For this review, take the finished solid that the model builds, in its own axes (mm). A direction names the side the tool comes from. Round coordinates to 2 decimals unless told otherwise and drop trailing zeros. Write each loop counter-clockwise with the first axis right and the second up, starting at its lowest first coordinate (ties: lowest second). Pieces come first, ordered by that corner, then holes. Notation, with made-up numbers: (69.5, 58.5) -> (120.5, 58.5) arc R21 cw to (120.5, 74.5) -> close; hole circle Ø3 at (-15.5, -10). An arc over 180 degrees is marked (long way). Write each question's results on one line, items separated by ' | '. Start each with the question number.
Item 1: The part is to be moulded in two halves that separate along X. For faces 1 (the cylindrical face through (6.06, -27.1, 20.28)), 2 (the flat face through (-17.5, 102, 20)), 3 (the cylindrical face through (5, -33, 1)), say which applies: +X half, -X half, draft (parallel to the pull), parting line (faces both ways), or undercut.
Item 2: Clearance check with flat-ended pins moving along their axes: pin 1 (0.6 mm diameter, centred on x = 4.5, z = 6.5, fed in from -Y); pin 2 (6 mm diameter, centred on y = 94.5, z = 24.5, fed in from +X); pin 3 (9 mm diameter, centred on x = 9.5, y = -49, fed in from +Z); pin 4 (3 mm diameter, centred on x = 15.5, y = 67, fed in from +Z). State where each tip first meets the part, or that it passes through.
Item 3: Add section A-A (y = 16). State the section outline as (x, z) points.
Item 4: Tool access review of faces 4 (the cylindrical face through (12.52, -46.26, 25.57)), 5 (the flat face through (5.2, -39, 20)), 6 (the cylindrical face through (4.9, -25.86, 20.28)): name each direction out of +Z, -Z, +X, -X, +Y, -Y from which nothing blocks a thin tool from reaching the whole face with its end or side.
Item 5: To check wall thickness, follow line 1 along Y through (x, z) = (13.5, 9.5); line 2 along X through (y, z) = (66.5, 38); line 3 along Y through (x, z) = (-2, 35.5). State the ranges of each line that lie inside material, in increasing order.
Item 6: Add section B-B (x = -5). State the section outline as (y, z) points.
from build123d import *

# Parameters (mm, degrees)
PAD_DEPTH    = 40
PAD001_DEPTH = 7
FILLET_R     = 3
FILLET001_R  = 5


with BuildPart() as part:
    # Sketch → Pad (new body)
    with BuildSketch(Plane.XY):
        Polygon((-17.5, 114), (17.5, 114), (17.5, 0), (24, 0), (24, -25), (4, -25), (4, -35), (5.2, -35), (5.2, -26.2), (25.2, -26.2), (25.2, 1.2), (18.7, 1.2), (18.7, 115.2), (-18.7, 115.2), (-18.7, 94), (-17.5, 94), align=None)
    extrude(amount=PAD_DEPTH)

    # Sketch001 → Pad001 (join, symmetric)
    with BuildSketch(Plane.XY.offset(20)):
        with BuildLine():
            Line((4, -35), (4, -55))
            ThreePointArc((4, -55), (7.7, -58.233631), (11.4, -55))
            Line((13.4, -45), (11.4, -55))
            Line((12.292308, -44.538462), (13.4, -45))
            Line((10.2, -55), (12.292308, -44.538462))
            ThreePointArc((5.2, -55), (7.7, -57.04951), (10.2, -55))
            Line((5.2, -55), (5.2, -35))
            Line((5.2, -35), (4, -35))
        make_face()
    extrude(amount=PAD001_DEPTH, both=True)

    # Fillet
    fillet_edges = [part.edges().sort_by_distance(p)[0] for p in [
        (24, -25, 20),
        (4, -25, 20),
        (17.5, 0, 20),
        (17.5, 114, 20),
        (-17.5, 114, 20),
        (24, 0, 20),
        (25.2, -26.2, 20),
        (25.2, 1.2, 20),
        (18.7, 115.2, 20),
        (5.2, -26.2, 20),
        (-18.7, 115.2, 20),
        (18.7, 1.2, 20),
    ]]
    fillet(fillet_edges, radius=FILLET_R)

    # Fillet001
    fillet001_edges = [part.edges().sort_by_distance(p)[0] for p in [
        (4.6, -35, 0),
        (4.6, -35, 13),
        (4.6, -35, 27),
        (4.6, -35, 40),
        (12.846154, -44.769231, 27),
        (12.846154, -44.769231, 13),
    ]]
    fillet(fillet001_edges, radius=FILLET001_R)


solid = part.part
Responses:
1) face 1: +X half | face 2: undercut | face 3: draft
2) pin 1: stops at y = -35 | pin 2: stops at x = 18.7 | pin 3: stops at z = 27 | pin 4: passes through
3) outline: (17.5, 0) -> (18.7, 0) -> (18.7, 40) -> (17.5, 40) -> close
4) face 4: +Z, +X | face 5: +Z, -Z | face 6: +Z, -Z, -X
5) line 1: y = -26.2 to -25, 114 to 115.2 | line 2: x = 17.5 to 18.7 | line 3: y = 114 to 115.2
6) outline: (114, 0) -> (115.2, 0) -> (115.2, 40) -> (114, 40) -> close
